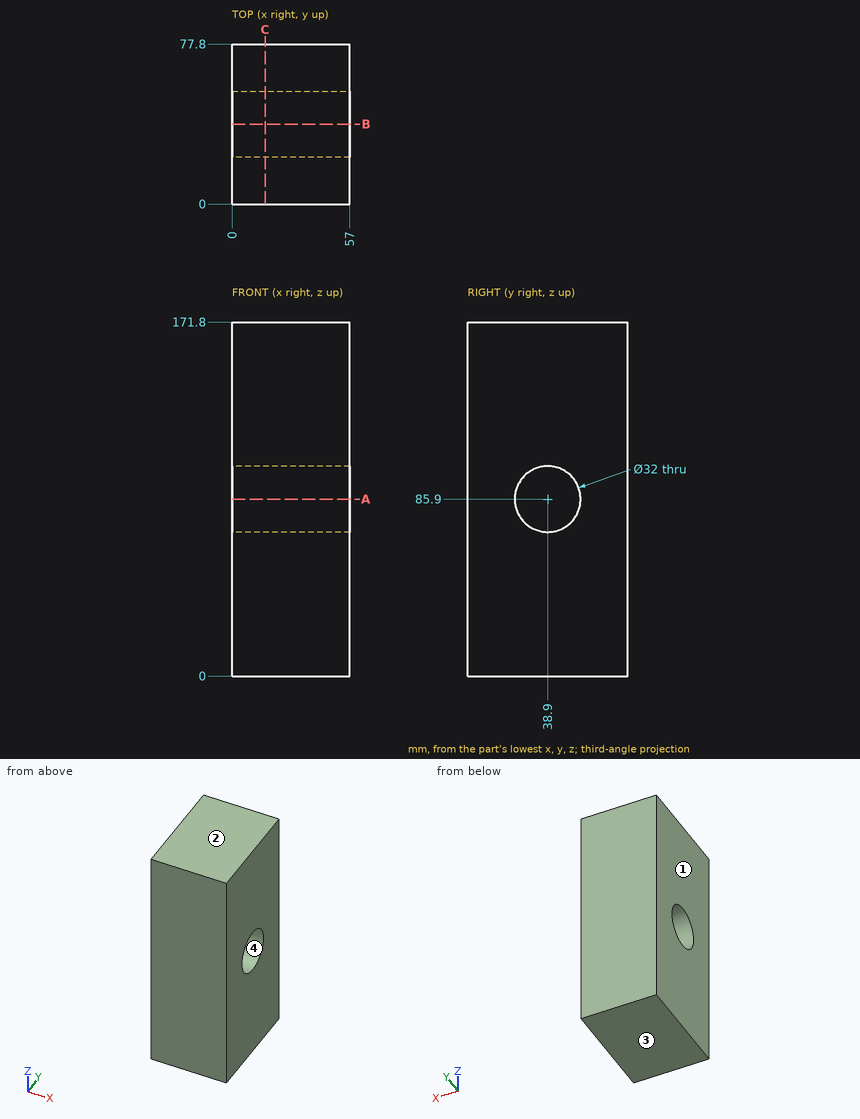
Print and shaded views of the part. All mm, measured from the part's lowest x, y and z. Round coordinates to 2 decimals unless told otherwise and drop trailing zeros. Write each loop counter-clockwise with the first axis right and the second up, starting at its lowest first coordinate (ties: lowest second). Pieces come first, ordered by that corner, then holes. Notation, with made-up numbers: (33.5, -6) -> (38.5, -6) arc R33 cw to (38.5, 30) -> close; hole circle Ø9 at (-1, -39). An arc over 180 degrees is marked (long way). Answer in a Markdown table with one row per item. Add a question column.
Item 1: Drop a flat-ended pin along its axis: pin 1 Ø19 at (y, z) = (38.9, 85.9) entering from -X. Give the stop position or say it passes through.
Item 2: Saw through at C-C, the plane x = 16. Write the cut outline in (y, z).
Item 3: Saw through at A-A, the plane z = 85.9. Write the cut outline in (x, y).
Item 4: Drill centre lines: line 1 (Y direction, x = 15, z = 85); line 2 (Z direction, x = 12, y = 38); line 3 (Z direction, x = 6, y = 25). Where is each one in solid material? Low to high. Write a range as from..to.
Item 5: Saw through at B-B, the plane y = 38.9. Write the cut outline in (x, z), then the cut area to 3 significant figures.
Item 6: Mould opens along Z. For the marked faces 1, 2, 3 and 4 say: pulls with the +Z half, pulls with the -Z half, needs draft (parallel to the pull), parting line crosses it, or undercut.
Findings below:
| question | item | result |
|---|---|---|
| 1 | pin 1 | passes through |
| 2 | outline | (0, 0) -> (77.8, 0) -> (77.8, 171.8) -> (0, 171.8) -> close; hole circle Ø32 at (38.9, 85.9) |
| 3 | outline | (0, 0) -> (57, 0) -> (57, 22.9) -> (0, 22.9) -> close; (0, 54.9) -> (57, 54.9) -> (57, 77.8) -> (0, 77.8) -> close |
| 4 | line 1 | y = 0..22.93, 54.87..77.8 |
| 4 | line 2 | z = 0..69.93, 101.87..171.8 |
| 4 | line 3 | z = 0..77.98, 93.82..171.8 |
| 5 | outline | (0, 0) -> (57, 0) -> (57, 69.9) -> (0, 69.9) -> close; (0, 101.9) -> (57, 101.9) -> (57, 171.8) -> (0, 171.8) -> close |
| 5 | area | 7,970 mm^2 |
| 6 | face 1 | needs draft |
| 6 | face 2 | pulls with the +Z half |
| 6 | face 3 | pulls with the -Z half |
| 6 | face 4 | undercut |
